```python
from build123d import *

# Parameters (mm, degrees)
F0_W     = 80.02039
F0_H     = 85.019648
F1_DEPTH = 25.4
F3_R     = 12.7
F2_DEPTH = 12.5


with BuildPart() as f1:
    # F0 (on Top) → F1 (new body)
    with BuildSketch(Plane.XY):
        with Locations((-0.330042, 3.939137)):
            Rectangle(F0_W, F0_H)
    extrude(amount=F1_DEPTH)

    # F3 (on face) → F2 (cut, symmetric)
    with BuildSketch(Plane.XY.offset(25.4)):
        Circle(F3_R)
    extrude(amount=F2_DEPTH, both=True, mode=Mode.SUBTRACT)


solid = f1.part
```
Geometry check sheet. Reference: the model listing, model coordinates, mm. A direction names the side the tool comes from. Give positions to 0.01 mm unless a question says otherwise; leave off trailing zeros. Order: outer loops, then holes, each group sorted by start corner. A loop starts at its lowest first (then second) coordinate and runs counter-clockwise, first axis right, second up.
1. Access from +Z, -Z, +X, -X, +Y, -Y to the whole of each face (thin tool, end or side, straight path). Record for faces 1 (the face through (-1, 46.449, 13)), 2 (the face through (-2.75, -12.4, 19.24)).
2. Section check C-C, the plane x = 0. Enter the section's corners in (y, z).
3. Section check A-A, the plane y = 0. Enter the section's corners in (x, z).
4. Release check for a two-part mould opening along X. For faces 3 (the face through (-1, 14, 25.4)), 4 (the face through (0, 0, 12.9)), 5 (the face through (39.68, 3, 13)) record: pulls with the +X half, pulls with the -X half, needs draft (parallel to the pull), parting line crosses it, or undercut.
5. Section check B-B, the plane z = 20.5. Enter the section's corners in (x, y), and give its area (3 significant figures).
6. Thickness scan on L1, parallel to Y at x = 0, z = 19.5; L2, parallel to Z at x = 9.5, y = 1; L3, parallel to X at y = -5, z = 14.25. Record the ranges inside material, lowest first.
Values follow:
1. face 1: +Z, -Z, +X, -X, +Y
1. face 2: +Z
2. outline: (-38.57, 0) - (46.45, 0) - (46.45, 25.4) - (12.7, 25.4) - (12.7, 12.9) - (-12.7, 12.9) - (-12.7, 25.4) - (-38.57, 25.4) - close
3. outline: (-40.34, 0) - (39.68, 0) - (39.68, 25.4) - (12.7, 25.4) - (12.7, 12.9) - (-12.7, 12.9) - (-12.7, 25.4) - (-40.34, 25.4) - close
4. face 3: needs draft
4. face 4: undercut
4. face 5: pulls with the +X half
5. outline: (-40.34, -38.57) - (39.68, -38.57) - (39.68, 46.45) - (-40.34, 46.45) - close; hole circle Ø25.4 at (0, 0)
5. area: 6,300 mm2
6. L1: y = -38.57 to -12.7, 12.7 to 46.45
6. L2: z = 0 to 12.9
6. L3: x = -40.34 to -11.67, 11.67 to 39.68
